The figure shows three views and two pictorial views of one solid part (mm, origin at its lowest corner). Answer the questions. Coordinates: 2 decimals unless noted, no trailing zeros. Write each loop counter-clockwise with the first axis right and the second up, starting at its lowest first coordinate (ties: lowest second). Pieces come first, ordered by that corner, then holes.
Item 1: Section D-D (y = 10.75) is taken. Give the vertices of the cut face in (x, z).
Item 2: Section C-C (z = 10.5) is taken. Give the vertices of the cut face in (x, y).
Item 3: Section A-A (y = 7) is taken. Give the vertices of the cut face in (x, z).
Item 4: Each of these flat-tipped pins is pushed along its axis until it touches: P1, Ø6, axis at x = 11, z = 17, coming from the +Y side; P2, Ø7, axis at x = 7, y = 7, coming from the +Z side; P3, Ø1.5, axis at x = 5.5, y = 7.5, coming from the -Z side. Where does it stop, or does it pass through?
Item 5: Determine the mould class of the marked faces 1, 2, 3 and 4 for opening direction Y: released by +Y, released by -Y, zero draft, split by the parting line, or undercut.
Item 6: Straight lines are drawn through the part: probe 1 along Y at (x, z) = (7, 17.25); probe 2 along Y at (x, z) = (7, 7.5); probe 3 along Z at (x, y) = (8.75, 7.5). For each, find the intervals that lie inside material, in ascending order.
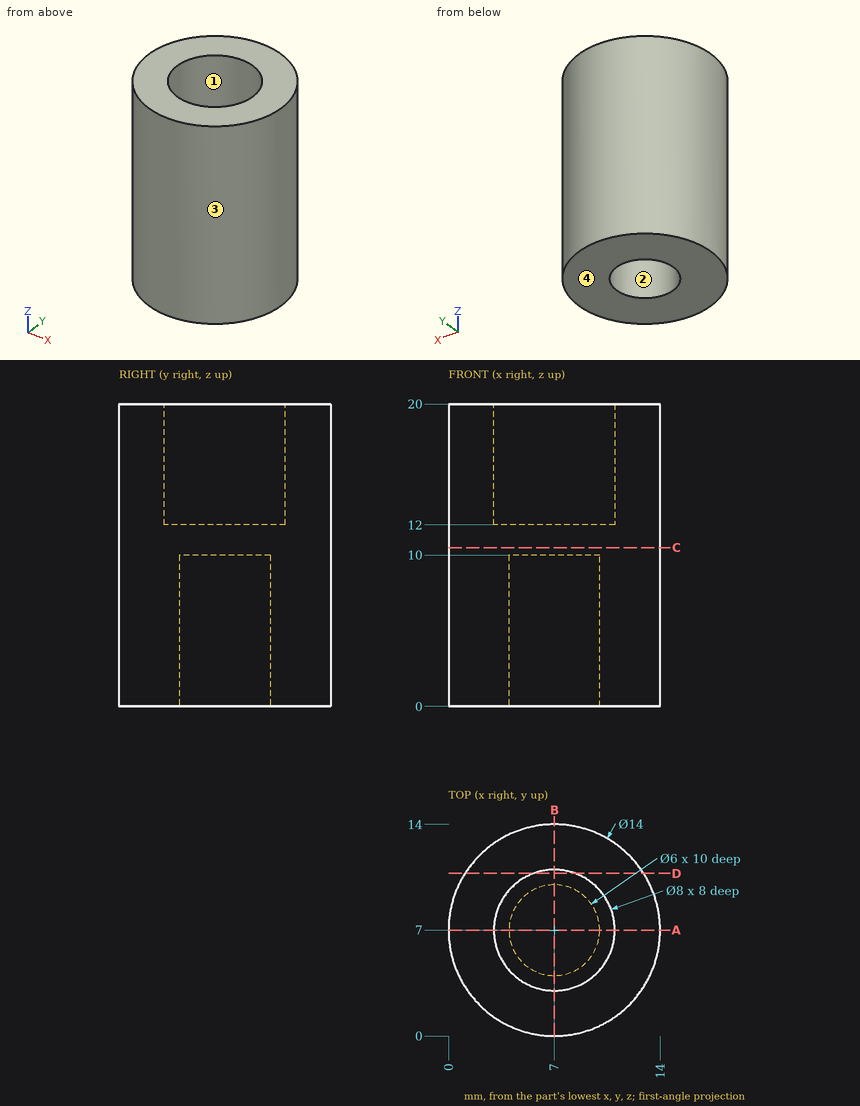
Established:
1. outline: (1.09, 0) - (12.91, 0) - (12.91, 20) - (8.39, 20) - (8.39, 12) - (5.61, 12) - (5.61, 20) - (1.09, 20) - close
2. outline: circle Ø14 at (7, 7)
3. outline: (0, 0) - (4, 0) - (4, 10) - (10, 10) - (10, 0) - (14, 0) - (14, 20) - (11, 20) - (11, 12) - (3, 12) - (3, 20) - (0, 20) - close
4. P1: stops at y = 13.93
4. P2: stops at z = 12
4. P3: stops at z = 10
5. face 1: undercut
5. face 2: undercut
5. face 3: split by the parting line
5. face 4: zero draft
6. probe 1: y = 0 to 3, 11 to 14
6. probe 2: y = 0 to 4, 10 to 14
6. probe 3: z = 10 to 12
